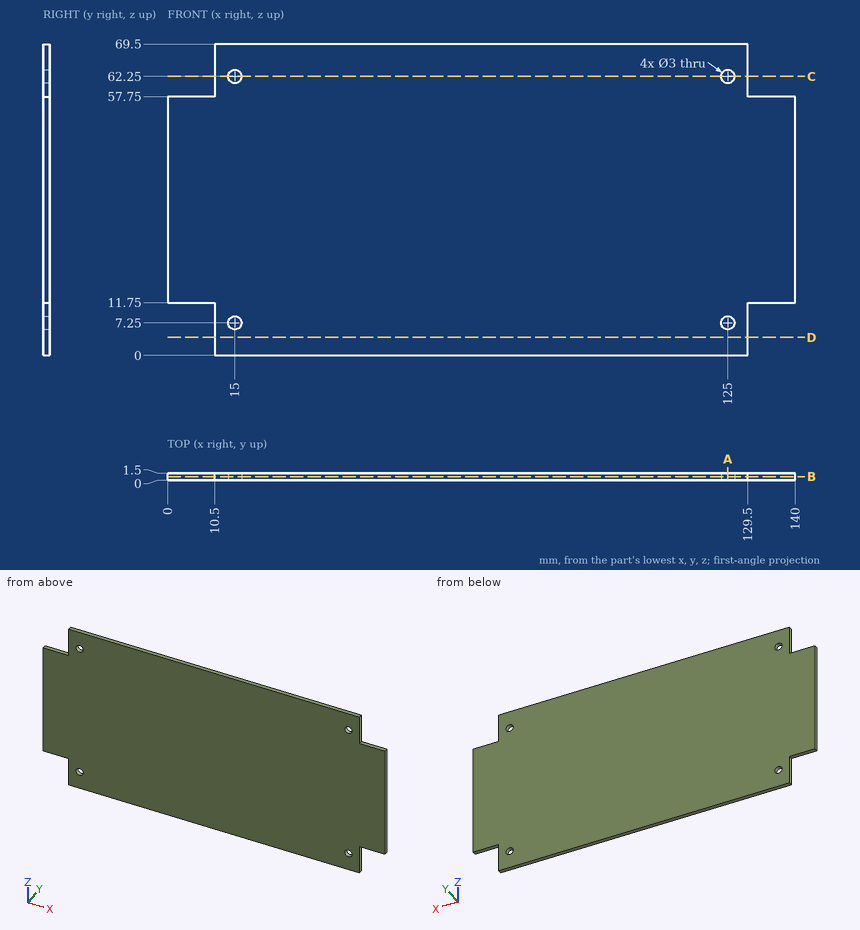
Could you check a few things on this drawing? It's one solid part, dimensions in mm from its lowest x, y, z. Round coordinates to 2 decimals unless told otherwise and drop trailing zeros. Order: outer loops, then holes, each group sorted by start corner. A loop starts at its lowest first (then second) coordinate and runs counter-clockwise, first axis right, second up. Notation, with made-up numbers: M 40,9.5 L 83,9.5 A18 ccw 83,18.5 Z; hole C -12,82.25 d2. An arc over 180 degrees is marked long. Return JSON: item names as keys, results as strings. Group by question number.
1. If we section it at A-A on x = 125: List the corners of the cut face in (y, z) for me, then the cut area to 4 significant figures.
2. If we section it at D-D on z = 4: List the corners of the cut face in (x, y) for me.
3. Please list where these lines run through material, in increasing order: probe 1 along Z at (x, y) = (125, 1.1); probe 2 along X at (y, z) = (1.2, 7.25); probe 3 along Z at (x, y) = (8, 0.7).
4. If we section it at C-C on z = 62.25: List the corners of the cut face in (x, y) for me.
5. If we section it at B-B on y = 0.8: List the corners of the cut face in (x, z) for me, then the cut area to 3 significant figures.
Reply:
{
 "1": {"outline": "M 0,0 L 1.5,0 L 1.5,5.75 L 0,5.75 Z; M 0,8.75 L 1.5,8.75 L 1.5,60.75 L 0,60.75 Z; M 0,63.75 L 1.5,63.75 L 1.5,69.5 L 0,69.5 Z", "area": "95.25 mm^2"},
 "2": {"outline": "M 10.5,0 L 129.5,0 L 129.5,1.5 L 10.5,1.5 Z"},
 "3": {"probe 1": "0 to 5.75, 8.75 to 60.75, 63.75 to 69.5", "probe 2": "10.5 to 13.5, 16.5 to 123.5, 126.5 to 129.5", "probe 3": "11.75 to 57.75"},
 "4": {"outline": "M 10.5,0 L 13.5,0 L 13.5,1.5 L 10.5,1.5 Z; M 16.5,0 L 123.5,0 L 123.5,1.5 L 16.5,1.5 Z; M 126.5,0 L 129.5,0 L 129.5,1.5 L 126.5,1.5 Z"},
 "5": {"outline": "M 0,11.75 L 10.5,11.75 L 10.5,0 L 129.5,0 L 129.5,11.75 L 140,11.75 L 140,57.75 L 129.5,57.75 L 129.5,69.5 L 10.5,69.5 L 10.5,57.75 L 0,57.75 Z; hole C 15,7.25 d3; hole C 15,62.25 d3; hole C 125,7.25 d3; hole C 125,62.25 d3", "area": "9,210 mm^2"}
}
